```python
from build123d import *

# Parameters (mm, degrees)
SKETCH_1_R      = 1.05
SKETCH_1_R_2    = 1.585
SKETCH_1_W      = 9
SKETCH_1_H      = 9
SKETCH_1_W_2    = 11
SKETCH_1_H_2    = 12
SKETCH_1_W_3    = 14
SKETCH_1_H_3    = 7
SKETCH_1_R_3    = 4
EXTRUDE_1_DEPTH = 2


with BuildPart() as part:
    # 草图1 → 凸台-拉伸1 (new body)
    with BuildSketch(Plane(origin=(0, 0, 0), x_dir=(1, 0, 0), z_dir=(0, 1, 0))):
        Polygon((70.16, 0), (0, 0), (0, -115), (99.16, -115), (99.16, -101), (94.16, -101), (94.16, -13), (99.16, -13), (99.16, 0), (88.16, 0), (88.16, -32), (70.16, -32), align=None)
        with Locations(Location((15.69, -113, 0), (0, 0, 270))):
            Circle(SKETCH_1_R, mode=Mode.SUBTRACT)
        with Locations(Location((22.16, -87.2, 0), (0, 0, 270))):
            Circle(SKETCH_1_R_2, mode=Mode.SUBTRACT)
        with Locations(Location((65.96, -95, 0), (0, 0, 270))):
            Circle(SKETCH_1_R, mode=Mode.SUBTRACT)
        with Locations(Location((66.66, -87.2, 0), (0, 0, 270))):
            Circle(SKETCH_1_R_2, mode=Mode.SUBTRACT)
        with Locations(Location((78.69, -113, 0), (0, 0, 270))):
            Circle(SKETCH_1_R, mode=Mode.SUBTRACT)
        with Locations(Location((90.66, -101.2, 0), (0, 0, 270))):
            Circle(SKETCH_1_R_2, mode=Mode.SUBTRACT)
        with Locations(Location((91.36, -95, 0), (0, 0, 270))):
            Circle(SKETCH_1_R, mode=Mode.SUBTRACT)
        Polygon((50.16, -83.5), (50.16, -77.5), (54.66, -77.5), (54.66, -83), (63.16, -83), (63.16, -93), (53.16, -93), (53.16, -83.5), align=None, mode=Mode.SUBTRACT)
        with Locations((78.66, -67.5)):
            Rectangle(SKETCH_1_W, SKETCH_1_H, mode=Mode.SUBTRACT)
        with Locations(Location((22.16, -27.46, 0), (0, 0, 270))):
            Circle(SKETCH_1_R_2, mode=Mode.SUBTRACT)
        with Locations((19.5, -15)):
            Rectangle(SKETCH_1_W_2, SKETCH_1_H_2, mode=Mode.SUBTRACT)
        with Locations(Location((15.69, -2, 0), (0, 0, 270))):
            Circle(SKETCH_1_R, mode=Mode.SUBTRACT)
        with Locations((50.16, -45.5)):
            Rectangle(SKETCH_1_W_3, SKETCH_1_H_3, mode=Mode.SUBTRACT)
        with Locations(Location((65.96, -54, 0), (0, 0, 270))):
            Circle(SKETCH_1_R, mode=Mode.SUBTRACT)
        with Locations(Location((56.66, -33.5, 0), (0, 0, 270))):
            Circle(SKETCH_1_R_3, mode=Mode.SUBTRACT)
        with Locations(Location((91.36, -54, 0), (0, 0, 270))):
            Circle(SKETCH_1_R, mode=Mode.SUBTRACT)
        with Locations(Location((66.66, -27.46, 0), (0, 0, 270))):
            Circle(SKETCH_1_R_2, mode=Mode.SUBTRACT)
        with Locations(Location((90.66, -13.2, 0), (0, 0, 270))):
            Circle(SKETCH_1_R_2, mode=Mode.SUBTRACT)
        with Locations(Location((8.12, -12.2, 0), (0, 0, 270))):
            Circle(SKETCH_1_R_2, mode=Mode.SUBTRACT)
        with Locations(Location((8.62, -38.06, 0), (0, 0, 270))):
            Circle(SKETCH_1_R_2, mode=Mode.SUBTRACT)
    extrude(amount=EXTRUDE_1_DEPTH)


solid = part.part
```
For this review, take the finished solid that the model builds, in its own axes (mm). Coordinates: 2 decimals unless noted, no trailing zeros. Loops run counter-clockwise (first coordinate to the right, second up) from the corner with the lowest first, then second, coordinate; pieces in that order, holes last.
1. Insertion check: P1, Ø0.6, axis at x = 79, y = 1, coming from the -Z side; P2, Ø0.6, axis at y = 1.5, z = 45, coming from the +X side. Each pin has a flat end and moves straight along its axis. Give the tip position at first contact, or say it passes through.
2. Add section C-C, the plane z = 27.46. Give the boundary of the cut face in (x, y) (3 decimals).
3. Add section A-A, the plane z = 47. Give the boundary of the cut face in (x, y).
4. Mouldability with a two-part tool opening along Z and no side actions: class faces 1 (the cylindrical face through (21.553, 0.986, 28.924)), 2 (the flat face through (49, 0, 57)) as +Z half, -Z half, draft (parallel to the pull), parting line (faces both ways), or undercut.
5. For line 1 (X direction, y = 1.75, z = 15); line 2 (Z direction, x = 56.5, y = 0.2); line 3 (X direction, y = 0.2, z = 64), list the stretches that pass through material, from the lowest coordinate up.
6. Add section B-B, the plane x = 22.16. Give the boundary of the cut face in (y, z) (3 decimals), then the cut area to 3 significant figures.
7. Add section D-D, the plane y = 1.7. Count the separate pieces of the cut face and the enclosed holes in it, then the cut area to 3 significant figures.
Result:
1. P1: stops at z = 32
1. P2: stops at x = 94.16
2. outline: (0, 0) - (20.575, 0) - (20.575, 2) - (0, 2) - close; (23.745, 0) - (65.075, 0) - (65.075, 2) - (23.745, 2) - close; (68.245, 0) - (70.16, 0) - (70.16, 2) - (68.245, 2) - close; (88.16, 0) - (94.16, 0) - (94.16, 2) - (88.16, 2) - close
3. outline: (0, 0) - (43.16, 0) - (43.16, 2) - (0, 2) - close; (57.16, 0) - (94.16, 0) - (94.16, 2) - (57.16, 2) - close
4. face 1: undercut
4. face 2: draft
5. line 1: x = 0 to 14, 25 to 70.16, 88.16 to 94.16
5. line 2: z = 0 to 29.5, 37.5 to 42, 49 to 83, 93 to 115
5. line 3: x = 0 to 74.16, 83.16 to 94.16
6. outline: (0, 0) - (2, 0) - (2, 9) - (0, 9) - close; (0, 21) - (2, 21) - (2, 25.875) - (0, 25.875) - close; (0, 29.045) - (2, 29.045) - (2, 85.615) - (0, 85.615) - close; (0, 88.785) - (2, 88.785) - (2, 115) - (0, 115) - close
6. area: 193 mm2
7. separate pieces: 1
7. enclosed holes: 20
7. area: 9,810 mm2
